```python
from build123d import *

# Parameters (mm, degrees)
SKETCH4_W           = 195.58
SKETCH4_H           = 76.2
SKETCH4_R           = 8.255
BOSS_EXTRUDE2_DEPTH = 2.54
SKETCH7_R           = 9.525
SKETCH7_W           = 76.2
SKETCH7_H           = 2.54
BOSS_EXTRUDE4_DEPTH = 2.54
SKETCH9_R           = 9.525
BOSS_EXTRUDE5_DEPTH = 2.54
SKETCH10_R          = 9.525
BOSS_EXTRUDE6_DEPTH = 2.54


with BuildPart() as part:
    # Sketch4 → Boss-Extrude2 (new body)
    with BuildSketch(Plane(origin=(0, 0, 0), x_dir=(1, 0, 0), z_dir=(0, 1, 0))):
        with Locations((97.79, 38.1)):
            Rectangle(SKETCH4_W, SKETCH4_H)
        with Locations((75.2856, 38.1)):
            Circle(SKETCH4_R, mode=Mode.SUBTRACT)
    extrude(amount=BOSS_EXTRUDE2_DEPTH)

    # Sketch7 → Boss-Extrude4 (add)
    with BuildSketch(Plane(origin=(195.58, 0, 0), x_dir=(0, 0, -1), z_dir=(1, 0, 0))):
        Polygon((69.85, 0), (0, 0), (0, -115.396245002), (0, -117.936245002), (76.2, -117.936245002), (76.2, -115.396245002), (69.85, -115.396245002), align=None)
        with Locations((38.1, -72.216245002)):
            Circle(SKETCH7_R, mode=Mode.SUBTRACT)
        with Locations((38.1, 1.27)):
            Rectangle(SKETCH7_W, SKETCH7_H)
    extrude(amount=BOSS_EXTRUDE4_DEPTH)

    # Sketch9 → Boss-Extrude5 (add)
    with BuildSketch(Plane(origin=(0, -117.936245002, 0), x_dir=(-1, 0, 0), z_dir=(0, -1, 0))):
        Polygon((-198.12, 0), (-195.58, 0), (0, 0), (0, 76.2), (-195.58, 76.2), (-198.12, 76.2), align=None)
        with Locations((-75.2856, 38.1)):
            Circle(SKETCH9_R, mode=Mode.SUBTRACT)
    extrude(amount=-BOSS_EXTRUDE5_DEPTH)

    # Sketch10 → Boss-Extrude6 (add)
    with BuildSketch(Plane.ZY):
        Polygon((0, 2.54), (0, 0), (0, -115.396245002), (0, -117.936245002), (-76.2, -117.936245002), (-76.2, -115.396245002), (-69.85, -115.396245002), (-69.85, 0), (-76.2, 0), (-76.2, 2.54), align=None)
        with Locations((-38.1, -72.216245002)):
            Circle(SKETCH10_R, mode=Mode.SUBTRACT)
    extrude(amount=BOSS_EXTRUDE6_DEPTH)


solid = part.part
```
Part model, mm, in its own coordinate system. A direction names the side the tool comes from. Coordinates: 2 decimals unless noted, no trailing zeros. Write each loop counter-clockwise with the first axis right and the second up, starting at its lowest first coordinate (ties: lowest second). Pieces come first, ordered by that corner, then holes.
Item 1: Slice it at B-B (x = 98.5). Write the cut outline in (y, z).
Item 2: Slice it at D-D (z = -38.1). Write the cut outline in (x, y).
Item 3: Probe line 1 (Y direction, x = 50.5, z = -25); line 2 (Y direction, x = 196, z = -38); line 3 (X direction, y = -24, z = -61). List the from-to ranges inside material, lowest first.
Item 4: Slice it at A-A (z = -59.5). Write the cut outline in (x, y).
Item 5: Mould opens along Z. For faces 4 (the face through (-2.54, -57, -29)), 5 (the face through (82.91, 1.25, -34.94)), 6 (the face through (98, -116, 0)) say: released by +Z, released by -Z, zero draft, split by the parting line, or undercut.
Item 6: Pin check, flat tips, straight feed: pin 1 (22 mm diameter, centred on y = -72.22, z = -38.1, fed in from -X); pin 2 (0.8 mm diameter, centred on x = -1.5, y = -77, fed in from -Z). Stop position of each tip, or through.
Item 7: Slice it at C-C (y = -28). Write the cut outline in (x, z).
Item 8: Which spindle directions (+Z, -Z, +X, -X, +Y, -Y) get a long thin tool onto all of the face, cutting with end or side? Do faces 1 (the face through (-1.252, -64.185, -32.979)), 2 (the face through (0, -57, -34)), 3 (the face through (66.2, -116.68, -40.96)). Say none if no direction does.
Results found:
1. outline: (-117.94, -76.2) - (-115.4, -76.2) - (-115.4, 0) - (-117.94, 0) - close; (0, -76.2) - (2.54, -76.2) - (2.54, 0) - (0, 0) - close
2. outline: (-2.54, -117.94) - (65.76, -117.94) - (65.76, -115.4) - (0, -115.4) - (0, -81.74) - (-2.54, -81.74) - close; (-2.54, -62.69) - (0, -62.69) - (0, 0) - (67.03, 0) - (67.03, 2.54) - (-2.54, 2.54) - close; (83.54, 0) - (195.58, 0) - (195.58, -62.69) - (198.12, -62.69) - (198.12, 2.54) - (83.54, 2.54) - close; (84.81, -117.94) - (198.12, -117.94) - (198.12, -81.74) - (195.58, -81.74) - (195.58, -115.4) - (84.81, -115.4) - close
3. line 1: y = -117.94 to -115.4, 0 to 2.54
3. line 2: y = -117.94 to -81.74, -62.69 to 2.54
3. line 3: x = -2.54 to 0, 195.58 to 198.12
4. outline: (-2.54, -117.94) - (198.12, -117.94) - (198.12, 2.54) - (-2.54, 2.54) - close; hole (0, -115.4) - (195.58, -115.4) - (195.58, 0) - (0, 0) - close
5. face 4: zero draft
5. face 5: undercut
5. face 6: released by +Z
6. pin 1: stops at x = -2.54
6. pin 2: stops at z = -69.85
7. outline: (-2.54, -69.85) - (0, -69.85) - (0, 0) - (-2.54, 0) - close; (195.58, -69.85) - (198.12, -69.85) - (198.12, 0) - (195.58, 0) - close
8. face 1: +X, -X
8. face 2: +Z, -Z
8. face 3: -Y
